The figure shows three views and two pictorial views of one solid part (mm, origin at its lowest corner). Answer the questions. A direction names the side the tool comes from. Round coordinates to 2 decimals unless told otherwise and drop trailing zeros. Order: outer loops, then holes, each group sorted by start corner. A loop starts at its lowest first (then second) coordinate and runs counter-clockwise, first axis right, second up. Notation, with made-up numbers: (20, 78) -> (64, 78) arc R24 cw to (64, 109) -> close; hole circle Ø2 at (-28, 73.25). An arc over 180 degrees is marked (long way). Return JSON: item names as keys, results as strings. Group by question number.
(1) The part is cut by section A-A (x = 7.5). Determine the outline of the cut face in (y, z).
(2) The part is cut by section C-C (z = 14.5). Determine the outline of the cut face in (x, y), plus the area to 3 significant figures.
(3) Consider line 1 (Z direction, x = 3.25, y = 13.75); line 2 (X direction, y = 7.75, z = 6); line 3 (X direction, y = 6.5, z = 25). Determine where each line is inside the solid, lowest interval first. Write a range as [from, to].
(4) The part is cut by section D-D (y = 11.25). Determine the outline of the cut face in (x, z), plus the area to 3 significant figures.
(5) Which of the six approach directions +Z, -Z, +X, -X, +Y, -Y give full straight-line access (tool end or side, diameter ignored) to the marked faces 1 and 2?
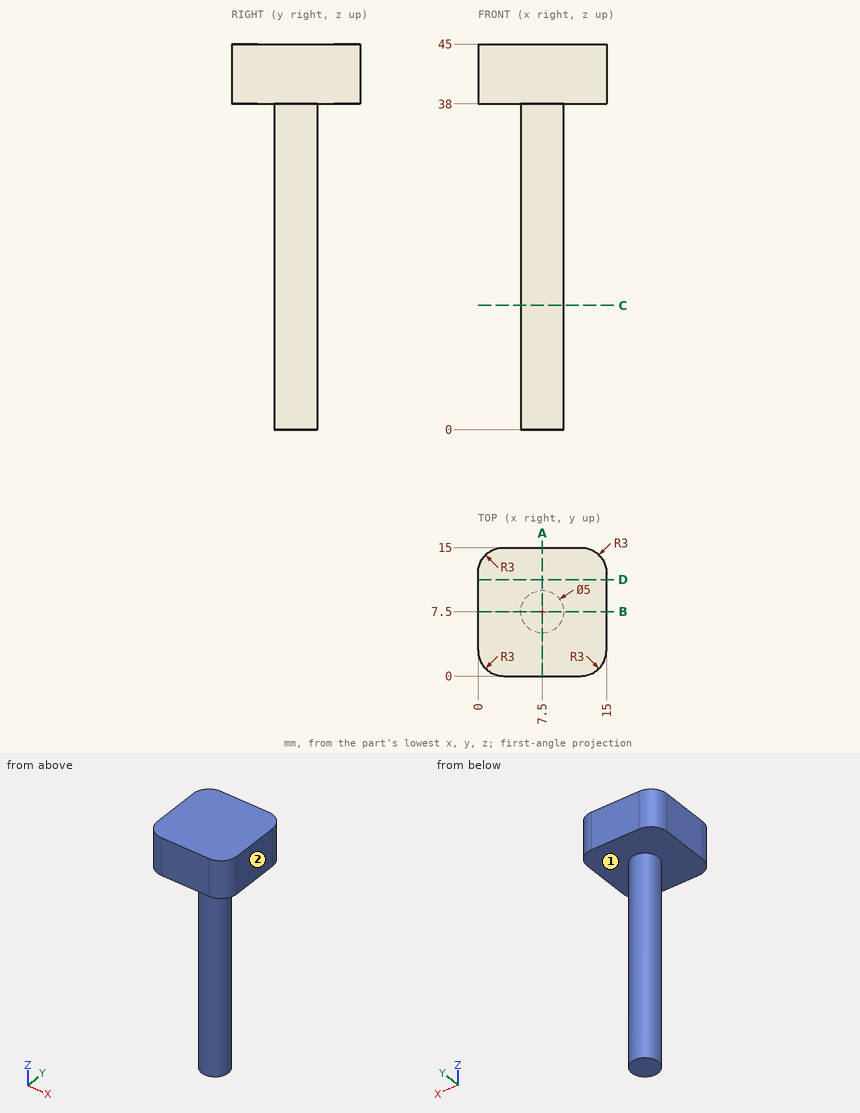
Answer below:
{
 "1": {"outline": "(0, 38) -> (5, 38) -> (5, 0) -> (10, 0) -> (10, 38) -> (15, 38) -> (15, 45) -> (0, 45) -> close"},
 "2": {"outline": "circle Ø5 at (7.5, 7.5)", "area": "19.6 mm²"},
 "3": {"line 1": "z = [38, 45]", "line 2": "x = [5.01, 9.99]", "line 3": "x = [5.21, 9.79]"},
 "4": {"outline": "(0, 38) -> (15, 38) -> (15, 45) -> (0, 45) -> close", "area": "105 mm²"},
 "5": {"face 1": "-Z", "face 2": "+Z, -Z, +X, +Y, -Y"}
}
